Verification items for the finished model (mm, model axes). A direction names the side the tool comes from. Coordinates: 2 decimals unless noted, no trailing zeros. Order: outer loops, then holes, each group sorted by start corner. A loop starts at its lowest first (then second) coordinate and runs counter-clockwise, first axis right, second up. Notation, with made-up numbers: (-31, 75) -> (24, 75) arc R14 ccw to (24, 98) -> close; hole circle Ø1 at (-1, -7.5). An arc over 180 degrees is marked (long way). Write item = value, one per line. Start each with the question number.
1. Thickness scan on line 1 along X through (y, z) = (0.5, -3); line 2 along Z through (x, y) = (-12, -0.5); line 3 along X through (y, z) = (5.5, -5). Record the ranges inside material, lowest first. Write a range as from..to.
2. Go/stop test with flat-tipped pins: P1, Ø0.5, axis at x = -2.5, z = 5.5, coming from the +Y side; P2, Ø3, axis at y = -4, z = -2, coming from the -X side; P3, Ø0.8, axis at x = 3, z = 7, coming from the -Y side. Record where each tip stops, or that it passes through.
3. Set-up check for faces 5 (the flat face through (-9, -3.844, 5)), 6 (the flat face through (-3, 0, 0)), 7 (the cylindrical face through (12.932, 5.362, 6.451)), 8 (the flat face through (3.2, 14.1, -43)): record each of +Z, -Z, +X, -X, +Y, -Y from which the full face is reachable in a straight line by a thin tool's end or side.
4. Release check for a two-part mould opening along X. For faces 1 (the cylindrical face through (-3.6, 1.4, 4.9)), 2 (the flat face through (3, -1, 10)), 3 (the flat face through (9, -3.844, 5)), 4 (the cylindrical face through (-14.985, 0.66, -20.037)) record: +X half, -X half, draft (parallel to the pull), parting line (faces both ways), or undercut.
5. Cross-section at B-B on z = -16.5. Record the cut outline in (x, y).
6. Cross-section at C-C on x = 11. Give the number of separate pieces and of enclosed holes in the cut face, plus the area to 3 significant figures.
Autodesk Fusion 360 part; units mm, degrees
sketch "Sketch1" plane through (0, 0, 0) normal (0, 0, 1) x (1, 0, 0)
  circle A0 centre (0, 0) radius 13
  circle A1 centre (0, 0) radius 14
  circle A2 centre (0, 0) radius 6 construction
  line L0 (-18, -0.0439) -> (20, -0.0439) construction
  line L1 (0, 17) -> (0, -15) construction
  circle A3 centre (-5.9998, -0.0439) radius 2.8
  circle A4 centre (5.9998, -0.0439) radius 2.8
  circle A5 centre (5.9998, -0.0439) radius 3.8
  circle A6 centre (-5.9998, -0.0439) radius 3.8
  line L2 (-18, -0.0439) -> (-18, 3.4561) construction
  line L3 (-18, 3.4561) -> (29, 3.4561) construction
  line L4 (-25, -0.3439) -> (-25, -3.8439) construction
  line L5 (-25, -3.8439) -> (28, -3.8439) construction
  line L6 (-4.52, 3.4561) -> (-12.5322, 3.4561)
  line L7 (-12.4187, -3.8439) -> (-5.9998, -3.8439)
  line L8 (7.4797, 3.4561) -> (12.5322, 3.4561)
  line L9 (5.9998, -3.8439) -> (12.4187, -3.8439)
  line L10 (6.6591, -0.3553) -> (-6.6591, -0.3553)
  line L11 (-6.6591, -0.3553) -> (-6.6591, 0.3553)
  line L12 (-6.6591, 0.3553) -> (6.6591, 0.3553)
  line L13 (6.6591, 0.3553) -> (6.6591, -0.3553)
  line L14 (6.6591, -0.3553) -> (-6.6591, 0.3553) construction
  line L15 (-6.6591, -0.3553) -> (6.6591, 0.3553) construction
  dimension "d1" = 26
  dimension "d2" = 28
  dimension "d3" = 12
  dimension "d4" = 5.6
  dimension "d5" = 5.6
  dimension "d6" = 7.6
  dimension "d7" = 7.6
  dimension "d8" = 3.5
  dimension "d9" = 47
  dimension "d10" = 3.5
  dimension "d11" = 53
  dimension "d12" = 0.7105
extrude "Extrude3" add sketch "Sketch1" along normal blind 10 contours A0 A5 L8 L9 | A0 A6 L6 L7 | A4 A5 L10 L12 | A3 A6 L6 L10 L12 | A1 picked at (2.5768, -0.5414) makes body 1
extrude "Extrude1" add sketch "Sketch1" along normal blind 4 separate body contours A0 A5 L8 L9 | A0 A6 L6 L7 | A4 A5 L10 L12 | A3 A6 L10 L12 | A1 picked at (2.5768, -0.5414) makes body 2 at (13.9304, -1.3939, 1.3333)
ref_plane "WorkPlane1" through (0, 0, 2) normal (0, 0, -1) x (-1, 0, 0)
sketch "Sketch2" plane through (0, 0, 2) normal (0, 0, -1) x (1, 0, 0)
  circle A0 centre (0, 0) radius 15
  circle A1 centre (0, 0) radius 14
  dimension "d16" = 30
  dimension "d17" = 28
extrude "Extrude2" add sketch "Sketch2" along normal blind 45 bodies 2 1
fillet "Fillet1" radius 0.3 1 edges at (-13.9849, 5.4242, -43) on bodies 2
fillet "Fillet2" radius 0.3 1 edges at (-13.0526, -5.0626, -43) on bodies 2
chamfer "Chamfer1" distance 1 angle 45 1 edges at (-13.0526, -5.0626, 2) on bodies 2
Worked out:
q1.line_1 = -14.99..-13.99, 13.99..14.99
q1.line_2 = 0..10
q1.line_3 = -13.96..-12.87, 12.87..13.96
q2.P1 = 13.82
q2.P2 = -14.79
q2.P3 = -13.76
q3.face_5 = +Z, -Z
q3.face_6 = -Z
q3.face_7 = +Z
q3.face_8 = -Z, +X, -X, +Y, -Y
q4.face_1 = undercut
q4.face_2 = draft
q4.face_3 = undercut
q4.face_4 = parting line
q5.outline = circle Ø30 at (0, 0); hole circle Ø28 at (0, 0)
q6.separate_pieces = 3
q6.enclosed_holes = 0
q6.area = 247 mm²
